CAD build for the part. Positions are in the model's coordinates, mm. Face numbers are marked on the shaded views. Coordinates: 2 decimals unless noted, no trailing zeros. Order: outer loops, then holes, each group sorted by start corner. A loop starts at its lowest first (then second) coordinate and runs counter-clockwise, first axis right, second up. Notation, with made-up numbers: M -21.5,-24 L 9.5,-24 A18 cw 9.5,4 Z; hole C 89.5,52.25 d5. An arc over 180 degrees is marked long. One line per item, written item: value.
from build123d import *

# Parameters (mm, degrees)
SKETCH1_R           = 50.8
SKETCH1_R_2         = 48.641
BOSS_EXTRUDE1_DEPTH = 114.3
SKETCH2_R           = 50.8
SKETCH2_R_2         = 48.641
SKETCH2_R_3         = 3.175
BOSS_EXTRUDE2_DEPTH = 3.175


with BuildPart() as part:
    # Sketch1 → Boss-Extrude1 (new body)
    with BuildSketch(Plane(origin=(0, 0, 0), x_dir=(1, 0, 0), z_dir=(0, 1, 0))):
        with Locations(Location((0, 0, 0), (0, 0, 270))):
            Circle(SKETCH1_R)
        with Locations(Location((0, 0, 0), (0, 0, 270))):
            Circle(SKETCH1_R_2, mode=Mode.SUBTRACT)
    extrude(amount=BOSS_EXTRUDE1_DEPTH)

    # Sketch2 → Boss-Extrude2 (add)
    with BuildSketch(Plane.XZ):
        with Locations(Location((0, 0, 0), (0, 0, 270))):
            Circle(SKETCH2_R)
        with Locations(Location((0, 0, 0), (0, 0, 90))):
            Circle(SKETCH2_R_2, mode=Mode.SUBTRACT)
        with Locations(Location((0, 0, 0), (0, 0, 90))):
            Circle(SKETCH2_R_2)
        with Locations(Location((38.1, 0, 0), (0, 0, 270))):
            Circle(SKETCH2_R_3, mode=Mode.SUBTRACT)
        with Locations(Location((-38.1, 0, 0), (0, 0, 270))):
            Circle(SKETCH2_R_3, mode=Mode.SUBTRACT)
    extrude(amount=BOSS_EXTRUDE2_DEPTH)


solid = part.part
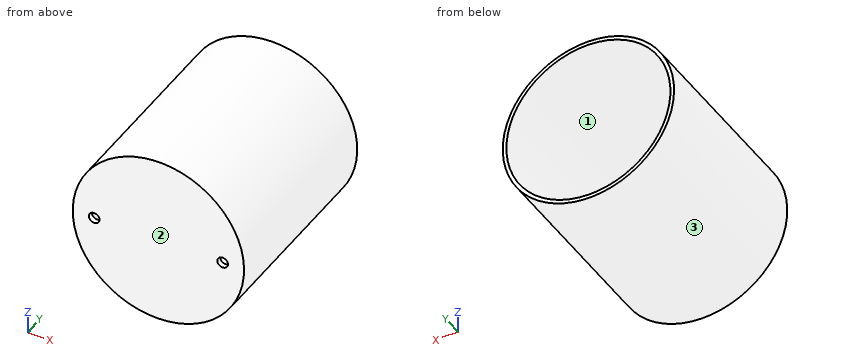
Q1. Mould opens along Z. For the marked faces 1, 2 and 3 say: released by +Z, released by -Z, zero draft, split by the parting line, or undercut.
Recorded:
face 1: undercut
face 2: zero draft
face 3: split by the parting line
Q2. Slice it at B-B (x = -38.1). List the corners of the cut face in (y, z) (3 decimals).
Recorded:
outline: M -3.175,-33.601 L 114.3,-33.601 L 114.3,-30.238 L 0,-30.238 L 0,-3.175 L -3.175,-3.175 Z; M -3.175,3.175 L 0,3.175 L 0,30.238 L 114.3,30.238 L 114.3,33.601 L -3.175,33.601 Z
Q3. Slice it at D-D (x = 0). List the corners of the cut face in (y, z) (3 decimals), plus the area to 3 significant figures.
Recorded:
outline: M -3.175,-50.8 L 114.3,-50.8 L 114.3,-48.641 L 0,-48.641 L 0,48.641 L 114.3,48.641 L 114.3,50.8 L -3.175,50.8 Z
area: 816 mm^2
Q4. Slice it at C-C (y = 27.5). List the corners of the cut face in (x, z).
Recorded:
outline: C 0,0 d101.6; hole C 0,0 d97.28
Q5. Slice it at A-A (z = 0). List the corners of the cut face in (x, y) (3 decimals).
Recorded:
outline: M -50.8,-3.175 L -41.275,-3.175 L -41.275,0 L -48.641,0 L -48.641,114.3 L -50.8,114.3 Z; M -34.925,-3.175 L 34.925,-3.175 L 34.925,0 L -34.925,0 Z; M 41.275,-3.175 L 50.8,-3.175 L 50.8,114.3 L 48.641,114.3 L 48.641,0 L 41.275,0 Z
Q6. Drill centre lines: line 1 along X through (y, z) = (-2.4, 0) (3 decimals); line 2 along X through (y, z) = (70.5, 0); line 3 along Y through (x, z) = (-1, 2.5) (3 decimals). Where is each one in solid material? Low to high.
Recorded:
line 1: x = -50.8 to -41.275, -34.925 to 34.925, 41.275 to 50.8
line 2: x = -50.8 to -48.64, 48.64 to 50.8
line 3: y = -3.175 to 0
Q7. Pin check, flat tips, straight feed: pin 1 Ø3 at (x, z) = (4.5, -33.5) entering from +Y; pin 2 Ø10 at (x, y) = (21.5, 99.5) entering from -Z; pin 3 Ø2 at (y, z) = (83, 39.5) entering from +X. Stop position of each tip, or through.
Recorded:
pin 1: stops at y = 0
pin 2: stops at z = -48.05
pin 3: stops at x = 33.14
